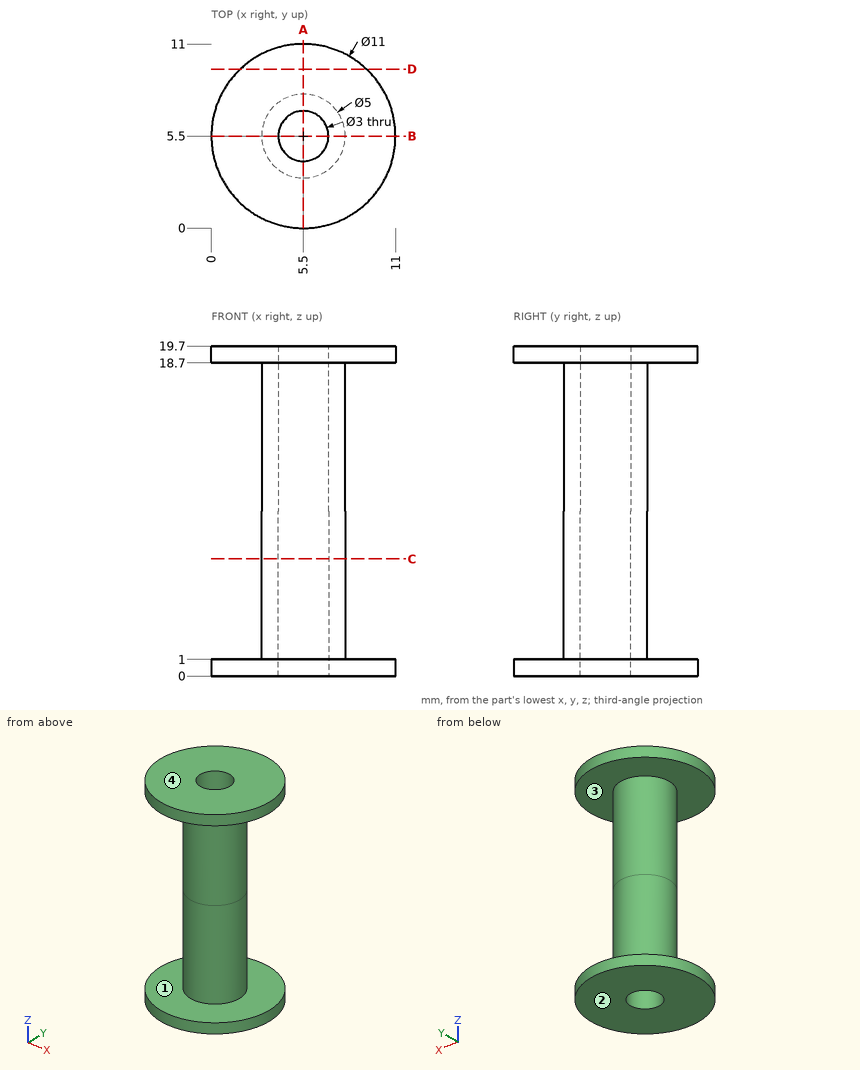
Source: three-view drawing plus pictorial views. Frame: mm from the lowest corner of the part. Coordinates: 2 decimals unless noted, no trailing zeros. Order: outer loops, then holes, each group sorted by start corner. A loop starts at its lowest first (then second) coordinate and runs counter-clockwise, first axis right, second up. Notation, with made-up numbers: M -17,0 L 33,0 A17 cw 33,17 Z; hole C 59,59 d10. An arc over 180 degrees is marked long. One line per question, with ' | ' between items.
Item 1: Pin query (flat end, axial travel): pin 1 (2 mm diameter, centred on x = 2.5, z = 7.5, fed in from +Y); pin 2 (2.5 mm diameter, centred on x = 5.5, y = 5.5, fed in from -Z); pin 3 (6 mm diameter, centred on x = 8, z = 5, fed in from +Y). Return the tip coordinate at first contact, or that it passes through.
Geometry results:
pin 1: stops at y = 7 | pin 2: passes through | pin 3: stops at y = 8
Item 2: Section A-A (x = 5.5). Output: boundary loops of the cut face in (y, z), then the cut area to 3 significant figures.
Geometry results:
outline: M 0,0 L 4,0 L 4,19.7 L 0,19.7 L 0,18.7 L 3,18.7 L 3,1 L 0,1 Z; M 7,0 L 11,0 L 11,1 L 8,1 L 8,18.7 L 11,18.7 L 11,19.7 L 7,19.7 Z | area: 51.4 mm^2
Item 3: Ray query, line 1 along Y through (x, z) = (5.5, 15); line 2 along Z through (x, y) = (6.25, 1.5); line 3 along X through (y, z) = (3.5, 15). Return the intervals inside material, ascending.
Geometry results:
line 1: y = 3 to 4, 7 to 8 | line 2: z = 0 to 1, 18.7 to 19.7 | line 3: x = 4 to 7
Item 4: Draft query along Z for the marked faces 1, 2, 3 and 4. Return one class per face: released by +Z, released by -Z, zero draft, split by the parting line, or undercut.
Geometry results:
face 1: undercut | face 2: released by -Z | face 3: undercut | face 4: released by +Z
Item 5: Section C-C (z = 7). Output: boundary loops of the cut face in (x, y).
Geometry results:
outline: C 5.5,5.5 d5; hole C 5.5,5.5 d3
Item 6: Section D-D (y = 9.5). Output: boundary loops of the cut face in (x, z), then the cut area to 3 significant figures.
Geometry results:
outline: M 1.73,0 L 9.27,0 L 9.27,1 L 1.73,1 Z; M 1.73,18.7 L 9.27,18.7 L 9.27,19.7 L 1.73,19.7 Z | area: 15.1 mm^2
